Can you work these out from the model? Positions are in its coordinate system, mm. A direction names the side the tool comes from. Round coordinates to 2 decimals unless told otherwise and drop trailing zeros. Order: outer loops, then holes, each group sorted by start corner. A loop starts at its lowest first (then second) coordinate and runs counter-clockwise, first axis right, second up. Notation, with made-up numbers: (17, -36) -> (40, -36) arc R16 cw to (40, -25) -> close; hole circle Ø9 at (-38.5, -13.75). An arc over 180 degrees is marked (long way). One line per item, written item: value.
```python
from build123d import *

# Parameters (mm, degrees)
CYLINDER085_R     = 1
CYLINDER085_DEPTH = 3.5
CYLINDER087_R     = 2
CYLINDER087_DEPTH = 3.5
CYLINDER086_R     = 7
CYLINDER086_DEPTH = 2.5
FILLET054_R       = 1.5


with BuildPart() as cylinder166:
    # Cylinder085 → Cylinder085 (new body)
    with BuildSketch(Plane(origin=(46, -9, 6), x_dir=(1, 0, 0), z_dir=(0, 0, 1))):
        Circle(CYLINDER085_R)
    extrude(amount=CYLINDER085_DEPTH)


with BuildPart() as cut111:
    # Cylinder087 → Cylinder087 (new body)
    with BuildSketch(Plane(origin=(46, -9, 6), x_dir=(1, 0, 0), z_dir=(0, 0, 1))):
        Circle(CYLINDER087_R)
    extrude(amount=CYLINDER087_DEPTH)

    # Cut111: cut Cylinder166
    add(cylinder166.part, mode=Mode.SUBTRACT)


with BuildPart() as fusion066:
    # Cylinder086 → Cylinder086 (new body)
    with BuildSketch(Plane(origin=(46, -9, 8), x_dir=(1, 0, 0), z_dir=(0, 0, 1))):
        Circle(CYLINDER086_R)
    extrude(amount=CYLINDER086_DEPTH)

    # Fillet054
    fillet054_edges = [fusion066.edges().sort_by_distance(p)[0] for p in [
        (39, -9, 10.5),
    ]]
    fillet(fillet054_edges, radius=FILLET054_R)

    # Fusion066: union Cut111
    add(cut111.part)


with BuildPart() as fusion066_1:
    # Fusion066 placement: moved
    add(fusion066.part.moved(Location((26, 0, 0))))


solid = fusion066_1.part
```
Q1. I want a section at B-B on z = 7.75. List the corners of the cut face in (x, y) for me, plus the area to 3 significant figures.
Answers below:
outline: circle Ø4 at (72, -9); hole circle Ø2 at (72, -9)
area: 9.42 mm^2
Q2. Please list where these lines run through material, in increasing order: line 1 along Y through (x, z) = (72, 7.05); line 2 along X through (y, z) = (-9, 6.4); line 3 along Z through (x, y) = (69.75, -10.5).
Answers below:
line 1: -11 to -10, -8 to -7
line 2: 70 to 71, 73 to 74
line 3: 8 to 10.5
Q3. I want a section at A-A on y = -9. List the corners of the cut face in (x, z) for me.
Answers below:
outline: (65, 8) -> (70, 8) -> (70, 6) -> (71, 6) -> (71, 8) -> (73, 8) -> (73, 6) -> (74, 6) -> (74, 8) -> (79, 8) -> (79, 9) arc R1.5 ccw to (77.5, 10.5) -> (66.5, 10.5) arc R1.5 ccw to (65, 9) -> close
Q4. Will these pins go through, and if not, where does the flat tip stop? pin 1 Ø2 at (x, z) = (74, 9) entering from +Y; pin 2 Ø3 at (x, y) = (72.5, -13.5) entering from -Z; pin 3 Ø2 at (x, z) = (66.5, 9) entering from -Y.
Answers below:
pin 1: y = -2.07
pin 2: z = 8
pin 3: y = -14.36
Q5. We'd pull the mould along Y, two halves only. Please class faces 3 (the face through (65.007, -8.692, 8.493)), 4 (the face through (73, -10, 6)), 5 (the face through (72, -9, 8)): released by +Y, released by -Y, zero draft, split by the parting line, or undercut.
Answers below:
face 3: split by the parting line
face 4: zero draft
face 5: undercut
Q6. I want a section at C-C on x = 72. List the corners of the cut face in (y, z) for me.
Answers below:
outline: (-16, 8) -> (-11, 8) -> (-11, 6) -> (-10, 6) -> (-10, 8) -> (-8, 8) -> (-8, 6) -> (-7, 6) -> (-7, 8) -> (-2, 8) -> (-2, 9) arc R1.5 ccw to (-3.5, 10.5) -> (-14.5, 10.5) arc R1.5 ccw to (-16, 9) -> close
Q7. I want a section at D-D on z = 8.65. List the corners of the cut face in (x, y) for me.
Answers below:
outline: circle Ø14 at (72, -9)
Q8. On a 3-axis mill with a long thin cutter (end or side, diameter ignored), from which of +Z, -Z, +X, -X, +Y, -Y can I reach the whole of each face in a straight line? I mean faces 1 (the face through (72, -9, 10.5)), 2 (the face through (71, -9, 7)). Say none if no direction works.
Answers below:
face 1: +Z, +X, -X, +Y, -Y
face 2: -Z
